Autodesk Inventor part; units mm, degrees
ref_plane "YZ Plane" through (0, 0, 0) normal (1, 0, 0) x (0, 1, 0)
ref_plane "XZ Plane" through (0, 0, 0) normal (0, 1, 0) x (-1, 0, 0)
ref_plane "XY Plane" through (0, 0, 0) normal (0, 0, 1) x (1, 0, 0)
sketch "Sketch5" plane through (0, 0, 0) normal (0, 0, 1) x (1, 0, 0)
  line L0 (-52.5, 30) -> (52.5, 30)
  line L1 (52.5, 30) -> (52.5, -30)
  line L2 (52.5, -30) -> (-52.5, -30)
  line L3 (-52.5, -30) -> (-52.5, 30)
  point P0 (0, 0)
  point P1 (0, 30)
  point P2 (52.5, 0)
  dimension "d8" = 60
  dimension "d9" = 105
extrude "Extrusion5" add sketch "Sketch5" along normal blind 30
sketch "Sketch6" plane through (0, 0, 30) normal (0, 0, 1) x (1, 0, 0)
  circle A0 centre (-27.5, -15) radius 4
  circle A1 centre (27.5, -15) radius 4
  line L0 (-52.5, -30) -> (52.5, -30)
  point P0 (0, 0)
  dimension "d12" = 55
  dimension "d13" = 27.5
  dimension "d14" = 8
  dimension "d39" = 15
hole "Hole1" at (-27.5, -15, 30) at (27.5, -15, 30) direction (0, 0, -1) diameter 9 end through all counterbore diameter 15 counterbore depth 9
sketch "Sketch7" plane through (-52.5, -30, 0) normal (-1, 0, 0) x (0, 0, 1)
  line L0 (0, 0) -> (30, 0)
  line L1 (0, 60) -> (30, 60)
  circle A0 centre (15, 50) radius 4
  circle A1 centre (15, 10) radius 4
  point P0 (0, 30)
  point P1 (15, 60)
  point P2 (15, 0)
  dimension "d22" = 40
  dimension "d23" = 20
  dimension "d24" = 8
hole "Hole2" at (-52.5, 20, 15) at (-52.5, -20, 15) direction (1, 0, 0) diameter 6.647 depth 18 tip angle 118
sketch "Sketch8" plane through (52.5, -30, 0) normal (1, 0, 0) x (0, 0, -1)
  circle A0 centre (-15, 10) radius 3.3235
  circle A1 centre (-15, 50) radius 3.3235
  circle A2 centre (-15, 10) radius 3.3235
  circle A3 centre (-15, 50) radius 3.3235
  point P0 (0, 30)
hole "Hole3" at (52.5, -20, 15) at (52.5, 20, 15) direction (-1, 0, 0) diameter 6.647 depth 18 tip angle 118
properties part number "BC-10012" material "Alumínio 7075"
Model file for the job. Use its own axes, mm. A direction names the side the tool comes from. Give positions to 0.01 mm unless a question says otherwise; leave off trailing zeros. Loops run counter-clockwise (first coordinate to the right, second up) from the corner with the lowest first, then second, coordinate; pieces in that order, holes last. Notation, with made-up numbers: (77, 1) - (110, 1) arc R16 ccw to (110, 10) - close; hole circle Ø3 at (-30.5, 61.5). An arc over 180 degrees is marked (long way). One line per item, written item: value. Start each with the question number.
1. Slice it at D-D (y = -8.5). List the corners of the cut face in (x, z), plus the area to 3 significant figures.
2. Pin check, flat tips, straight feed: pin 1 (8 mm diameter, centred on x = -27.5, y = -15, fed in from +Z); pin 2 (5.5 mm diameter, centred on y = 20, z = 15, fed in from +X); pin 3 (4 mm diameter, centred on y = -20, z = 15, fed in from -X). Stop position of each tip, or through.
3. Slice it at A-A (x = -27.5). List the corners of the cut face in (y, z).
4. Probe L1, parallel to Y at x = -45.75, z = 15; L2, parallel to X at y = -15, z = 23.75; L3, parallel to X at y = -15, z = 14.5. List the from-to ranges inside material, lowest first. Write a range as from..to.
5. Slice it at B-B (z = 10.5). List the corners of the cut face in (x, y).
6. Slice it at C-C (x = 40.5). List the corners of the cut face in (y, z), plus the area to 3 significant figures.
7. Which spindle directions (+Z, -Z, +X, -X, +Y, -Y) get a long thin tool onto all of the face, cutting with end or side? Do faces 1 (the cylindrical face through (-43.37, 17.2, 16.79)), 2 (the cylindrical face through (27.302, -10.504, 10.353)), 3 (the flat face through (-1, 0, 0)), 4 (the cylindrical face through (43.37, -22.8, 13.21)), 5 (the flat face through (27, -20, 21)). Say none if no direction does.
8. Pull direction X, two halves, no side cores. Call faces 6 (the cylindrical face through (34.82, -13.37, 25.44)), 7 (the cylindrical face through (-20.18, -13.37, 25.44)), 8 (the cylindrical face through (-43.37, -22.8, 16.79)), 9 (the conical face through (-32.85, -19.97, 14.42)): pulls with the +X half, pulls with the -X half, needs draft (parallel to the pull), parting line crosses it, or undercut.
Solution:
1. outline: (-52.5, 0) - (52.5, 0) - (52.5, 30) - (31.24, 30) - (31.24, 21) - (23.76, 21) - (23.76, 30) - (-23.76, 30) - (-23.76, 21) - (-31.24, 21) - (-31.24, 30) - (-52.5, 30) - close
1. area: 3,020 mm^2
2. pin 1: passes through
2. pin 2: stops at x = 34.16
2. pin 3: stops at x = -33.7
3. outline: (-30, 0) - (-19.5, 0) - (-19.5, 21) - (-22.5, 21) - (-22.5, 30) - (-30, 30) - close; (-10.5, 0) - (30, 0) - (30, 30) - (-7.5, 30) - (-7.5, 21) - (-10.5, 21) - close
4. L1: y = -30..-23.32, -16.68..16.68, 23.32..30
4. L2: x = -52.5..-35, -20..20, 35..52.5
4. L3: x = -52.5..-32, -23..23, 32..52.5
5. outline: (-52.5, -30) - (52.5, -30) - (52.5, 30) - (-52.5, 30) - close; hole circle Ø9 at (-27.5, -15); hole circle Ø9 at (27.5, -15)
6. outline: (-30, 0) - (30, 0) - (30, 30) - (-30, 30) - close; hole circle Ø6.65 at (-20, 15); hole circle Ø6.65 at (20, 15)
6. area: 1,730 mm^2
7. face 1: -X
7. face 2: +Z, -Z
7. face 3: -Z, +X, -X, +Y, -Y
7. face 4: +X
7. face 5: +Z
8. face 6: undercut
8. face 7: undercut
8. face 8: needs draft
8. face 9: pulls with the -X half
